Read the model definition and answer for the solid it produces. Units are mm, in the model's axes. Face numbers are marked on the shaded views. A direction names the side the tool comes from. Coordinates: 2 decimals unless noted, no trailing zeros. Write each loop counter-clockwise with the first axis right and the second up, starting at its lowest first coordinate (ties: lowest second). Pieces come first, ordered by that corner, then holes.
(1) Given pin 1 (12 mm diameter, centred on x = 0, y = 14, fed in from -Z); pin 2 (0.7 mm diameter, centred on y = 1, z = 7, fed in from +X); pin 3 (6 mm diameter, centred on x = 7.5, z = 13.5, fed in from -Y); pin 4 (1.8 mm diameter, centred on y = 0.5, z = 3, fed in from -X), each flat-ended and moving along its own axis, determine where each tip first touches the part or whether it passes through.
(2) The part is cut by section A-A, the plane y = 12.2. Determine the outline of the cut face in (x, z).
(3) The part is cut by section C-C, the plane z = -0.5. Determine the outline of the cut face in (x, y), and give its area (3 significant figures).
(4) Which of the six approach directions +Z, -Z, +X, -X, +Y, -Y give full straight-line access (tool end or side, diameter ignored) to the marked faces 1, 2, 3, 4 and 5?
(5) The part is cut by section B-B, the plane x = 0. Determine the outline of the cut face in (y, z), and give its area (3 significant figures).
(6) The part is cut by section D-D, the plane x = -3. Determine the outline of the cut face in (y, z), and give its area (3 significant figures).
(7) Straight lines are drawn through the part: line 1 along Z through (x, y) = (8.25, 2.5); line 2 along X through (y, z) = (12.2, 0.25); line 3 along Y through (x, z) = (0, 12). For each, find the intervals that lie inside material, in ascending order.
(8) Determine the mould class of the marked faces 6, 7 and 8 for opening direction Z: pulls with the +Z half, pulls with the -Z half, needs draft (parallel to the pull), parting line crosses it, or undercut.
Autodesk Inventor part; units mm, degrees
ref_plane "YZ Plane" through (0, 0, 0) normal (1, 0, 0) x (0, 1, 0)
ref_plane "XZ Plane" through (0, 0, 0) normal (0, 1, 0) x (-1, 0, 0)
ref_plane "XY Plane" through (0, 0, 0) normal (0, 0, 1) x (1, 0, 0)
sketch "Skizze2" plane through (0, 0, 0) normal (0, 0, 1) x (1, 0, 0)
  line L0 (2.4, 0) -> (2.4, 7)
  line L1 (-2.4, 0) -> (-2.4, 7)
  line L2 (0, 0) -> (2.4, 0) construction
  line L3 (-2.4, 7) -> (2.4, 7)
  line L4 (-2.4, 0) -> (-4.6, 0)
  line L5 (2.4, 0) -> (4.6, 0)
  arc A0 (-4.6, 0) -> (4.6, 0) centre (0, 4.29) ccw
  point P0 (0, -2)
  dimension "d0" = 7
  dimension "d1" = 4.8
  dimension "d2" = 2.4
  dimension "d3" = 2.2
  dimension "d4" = 2
extrude "Extrusion1" add sketch "Skizze2" along normal blind 15
sketch "Skizze3" plane through (0, 0, 15) normal (0, 0, 1) x (1, 0, 0)
  line L0 (-2.4, 0) -> (-2.4, 2.2) construction
  line L1 (-2.4, 2.2) -> (-10, 2.2)
  line L2 (-2.4, 2.2) -> (10, 2.2)
  line L3 (-10, 2.2) -> (10, 2.2)
  line L4 (10, 2.2) -> (10, 7)
  line L5 (10, 7) -> (-10, 7)
  line L6 (-10, 7) -> (-10, 2.2)
  line L7 (-10, 7) -> (10, 7)
  line L8 (10, 7) -> (10, 22.2)
  line L9 (10, 22.2) -> (-10, 22.2)
  line L10 (-10, 22.2) -> (-10, 7)
  point P0 (0, 0)
  point P1 (2.4, 7)
  dimension "d7" = 2.2
  dimension "d8" = 20
  dimension "d9" = 10
  dimension "d10" = 20
  dimension "d39" = 20
extrude "Extrusion2" add sketch "Skizze3" against normal blind 5
sketch "Skizze15" plane through (0, 0, 15) normal (0, 0, 1) x (1, 0, 0)
  circle A0 centre (0, 12.2) radius 7.5
  line L0 (-10, 22.2) -> (-10, 2.2)
  line L1 (10, 22.2) -> (-10, 22.2)
  point P0 (0, 0)
  dimension "d40" = 15
  dimension "d41" = 10
  dimension "d42" = 10
extrude "Extrusion12" cut sketch "Skizze15" against normal blind 5
sketch "Skizze16" plane through (0, 0, 0) normal (0, 0, -1) x (-1, 0, 0)
  line L0 (-10, 2.2) -> (-2.4, 2.2)
  line L1 (10, 22.2) -> (10, 2.2)
  line L2 (-10, 2.2) -> (10, 2.2)
  line L3 (10, 2.2) -> (10, 22.2)
  line L4 (10, 22.2) -> (-10, 22.2)
  line L5 (-10, 22.2) -> (-10, 2.2)
  point P0 (0, 0)
  point P1 (10, 2.2)
extrude "Extrusion13" cut sketch "Skizze16" against normal blind 10
ref_plane "Arbeitsebene3" through (0, 0, 7.5) normal (0, 0, -1) x (-1, 0, 0)
mirror "Spiegeln2" about plane through (0, 0, 7.5) normal (0, 0, -1) of "Extrusion2", "Extrusion12"
sketch "Skizze18" plane through (0, 0, 7.5) normal (0, 0, -1) x (-1, 0, 0)
  line L0 (10, 2.2) -> (10, 22.2)
  line L1 (-10, 22.2) -> (-10, 2.2)
  line L2 (10, 2.2) -> (-10, 2.2)
  line L3 (-10, 2.2) -> (-10, 22.2)
  line L4 (-10, 22.2) -> (10, 22.2)
  line L5 (10, 22.2) -> (10, 2.2)
  point P0 (0, 0)
  point P1 (-10, 2.2)
extrude "Extrusion14" cut sketch "Skizze18" along normal mid plane 5.2
sketch "Skizze19" plane through (0, 0, 15) normal (0, 0, 1) x (1, 0, 0)
  circle A0 centre (0, 12.2) radius 7.5
  line L0 (-2.4, 2.2) -> (-2.4, 0)
  line L1 (-2.4, 0) -> (-4.6, 0)
  arc A1 (-4.6, 0) -> (4.6, 0) centre (0, 4.29) ccw
  line L2 (4.6, 0) -> (2.4, 0)
  line L3 (2.4, 0) -> (2.4, 2.2)
  line L4 (2.4, 2.2) -> (10, 2.2)
  line L5 (10, 2.2) -> (10, 22.2)
  line L6 (10, 22.2) -> (-10, 22.2)
  line L7 (-10, 22.2) -> (-10, 2.2)
  line L8 (-10, 2.2) -> (-2.4, 2.2)
  point P0 (0, 0)
extrude "Extrusion15" add sketch "Skizze19" along normal blind 2.5
mirror "Spiegeln3" about plane through (0, 0, 7.5) normal (0, 0, -1) of "Extrusion15"
ref_plane "Arbeitsebene4" through (0, 0, 7.5) normal (0, 0, -1) x (-1, 0, 0)
properties part number "Connector MiniTec"
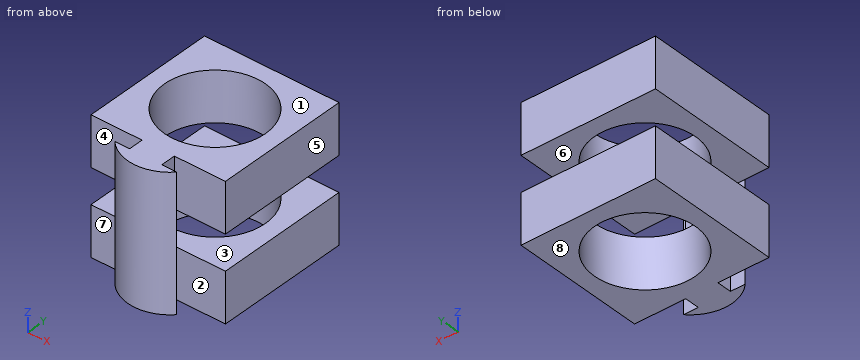
Computed:
1. pin 1: stops at z = -2.5
1. pin 2: stops at x = 2.4
1. pin 3: stops at y = -0.1
1. pin 4: stops at x = -4.6
2. outline: (-10, -2.5) - (-7.5, -2.5) - (-7.5, 4.9) - (-10, 4.9) - close; (-10, 10.1) - (-7.5, 10.1) - (-7.5, 17.5) - (-10, 17.5) - close; (7.5, -2.5) - (10, -2.5) - (10, 4.9) - (7.5, 4.9) - close; (7.5, 10.1) - (10, 10.1) - (10, 17.5) - (7.5, 17.5) - close
3. outline: (-10, 2.2) - (-2.4, 2.2) - (-2.4, 0) - (-4.6, 0) arc R6.29 ccw to (4.6, 0) - (2.4, 0) - (2.4, 2.2) - (10, 2.2) - (10, 22.2) - (-10, 22.2) - close; hole circle Ø15 at (0, 12.2)
3. area: 247 mm2
4. face 1: +Z, +X, -X, +Y, -Y
4. face 2: +Z, -Z, +X
4. face 3: +X, -X, +Y
4. face 4: +Z, -Z, -X
4. face 5: +Z, -Z, +X, +Y, -Y
5. outline: (-2, -2.5) - (4.7, -2.5) - (4.7, 4.9) - (2.2, 4.9) - (2.2, 10.1) - (4.7, 10.1) - (4.7, 17.5) - (-2, 17.5) - close; (19.7, -2.5) - (22.2, -2.5) - (22.2, 4.9) - (19.7, 4.9) - close; (19.7, 10.1) - (22.2, 10.1) - (22.2, 17.5) - (19.7, 17.5) - close
5. area: 158 mm2
6. outline: (-1.24, -2.5) - (0, -2.5) - (0, 17.5) - (-1.24, 17.5) - close; (2.2, -2.5) - (5.33, -2.5) - (5.33, 4.9) - (2.2, 4.9) - close; (2.2, 10.1) - (5.33, 10.1) - (5.33, 17.5) - (2.2, 17.5) - close; (19.07, -2.5) - (22.2, -2.5) - (22.2, 4.9) - (19.07, 4.9) - close; (19.07, 10.1) - (22.2, 10.1) - (22.2, 17.5) - (19.07, 17.5) - close
6. area: 117 mm2
7. line 1: z = -2.5 to 4.9, 10.1 to 17.5
7. line 2: x = -10 to -7.5, 7.5 to 10
7. line 3: y = -2 to 4.7, 19.7 to 22.2
8. face 6: undercut
8. face 7: needs draft
8. face 8: pulls with the -Z half
